Can you work these out from the model? Positions are in its coordinate system, mm. A direction names the side the tool comes from. Round coordinates to 2 decimals unless told otherwise and drop trailing zeros. Order: outer loops, then holes, each group sorted by start corner. A loop starts at its lowest first (then second) coordinate and runs counter-clockwise, first axis right, second up. Notation, with made-up numbers: (29, 75) -> (53, 75) arc R33 cw to (53, 103) -> close; hole circle Ø9 at (64, 8.25). An arc over 180 degrees is marked (long way). Use a Markdown table: item, result. Add a question column.
Q1. I need wall thicknesses on line 1 along Z through (x, y) = (-62, 4.2); line 2 along X through (y, z) = (1.65, -12.5); line 3 along X through (y, z) = (1.45, -61). Which ranges of each line are inside material? Lowest first, please. Write a range as [from, to].
Q2. If we section it at D-D on x = -42: List the corners of the cut face in (y, z) for me, plus the area to 3 significant figures.
Q3. If we section it at A-A on z = -37.5: List the corners of the cut face in (x, y) for me, plus the area to 3 significant figures.
Q4. If we section it at B-B on x = -87: List the corners of the cut face in (y, z) for me, plus the area to 3 significant figures.
Q5. We'd pull the mould along X, two halves only. Please class faces 1 (the face through (-44.027, 3.042, -39.359)), 2 (the face through (-103, 3, -74)), 3 (the face through (-33, 3, -2)): +X half, -X half, draft (parallel to the pull), parting line (faces both ways), or undercut.
Q6. If we section it at C-C on y = 1.65: List the corners of the cut face in (x, z) for me.
Q7. For faces 4 (the face through (-75, 3, -62)), 5 (the face through (-105, 3, -37)), 6 (the face through (-84.25, 3, -65)), which set-ups out of +Z, -Z, +X, -X, +Y, -Y let a thin tool reach every point of the face, with its end or its side?
Q8. I'm going to push flat-ended pins straight in: pin 1 Ø5 at (x, z) = (-62, -37.5) entering from +Y; pin 2 Ø3 at (y, z) = (3, -61) entering from +X. Where does each tip first touch, or does it pass through?
Autodesk Inventor part; units mm, degrees
ref_plane "YZ Plane" through (0, 0, 0) normal (1, 0, 0) x (0, 1, 0)
ref_plane "XZ Plane" through (0, 0, 0) normal (0, 1, 0) x (-1, 0, 0)
ref_plane "XY Plane" through (0, 0, 0) normal (0, 0, 1) x (1, 0, 0)
sketch "Sketch1" plane through (0, 0, 0) normal (0, 1, 0) x (-1, 0, 0)
  line L0 (0, 0) -> (105, 0)
  line L1 (105, 0) -> (105, -50)
  line L2 (105, -50) -> (0, -50)
  line L3 (0, -50) -> (0, 0)
  line L4 (0, 0) -> (0, -16.6667)
  line L5 (0, -16.6667) -> (11, -16.6667)
  dimension "d0" = 105
  dimension "d1" = 50
  dimension "d2" = 16.6667
  dimension "d3" = 11
extrude "Extrusion1" add sketch "Sketch1" along normal blind 6
sketch "Sketch3" plane through (0, 6, 0) normal (0, 1, 0) x (1, 0, 0)
  circle A0 centre (-20, 12.5) radius 2.75
  line L0 (0, 0) -> (0, 50)
  line L1 (-105, 0) -> (0, 0)
  circle A1 centre (-20, 37.5) radius 2.75
  dimension "d21" = 5.5
  dimension "d22" = 20
  dimension "d23" = 12.5
  dimension "d26" = 25
extrude "Extrusion3" cut sketch "Sketch3" against normal through all
sketch "Sketch4" plane through (0, 6, 0) normal (0, 1, 0) x (1, 0, 0)
  circle A0 centre (-20, 12.5) radius 2.75
  line L0 (-20, 12.5) -> (-75, 12.5)
  line L1 (-75, 12.5) -> (-90, 12.5) construction
  line L2 (-75, 15.25) -> (-90, 15.25)
  line L3 (-90, 9.75) -> (-75, 9.75)
  arc A1 (-75, 9.75) -> (-75, 15.25) centre (-75, 12.5) ccw
  arc A2 (-90, 15.25) -> (-90, 9.75) centre (-90, 12.5) ccw
  point P0 (0, 0)
  point P1 (-82.5, 12.5)
  dimension "d33" = 55
  dimension "d34" = 15
  dimension "d35" = 5.5
extrude "Extrusion4" cut sketch "Sketch4" against normal through all contours A1 L3 A2 L2
pattern_linear "Rectangular Pattern2" count 2 spacing 25 along (0, 0, -1) of "Extrusion4"
sketch "Sketch5" plane through (0, 0, -50) normal (0, 0, -1) x (-1, 0, 0)
  line L0 (105, 0) -> (105, 6)
  line L1 (105, 0) -> (0, 0)
  line L2 (105, 6) -> (75, 6)
  line L3 (75, 6) -> (75, 0)
  line L4 (75, 0) -> (105, 0)
  line L5 (105, 0) -> (105, 6)
  dimension "d45" = 30
extrude "Extrusion5" add sketch "Sketch5" along normal blind 25
sketch "Sketch6" plane through (0, 6, 0) normal (0, 1, 0) x (1, 0, 0)
  line L0 (-87, 60.5) -> (-87, 70.5) construction
  line L1 (-84.25, 60.5) -> (-84.25, 70.5)
  line L2 (-89.75, 70.5) -> (-89.75, 60.5)
  arc A0 (-89.75, 60.5) -> (-84.25, 60.5) centre (-87, 60.5) ccw
  arc A1 (-84.25, 70.5) -> (-89.75, 70.5) centre (-87, 70.5) ccw
  line L3 (-75, 50) -> (-75, 75)
  arc A2 (-90, 40.25) -> (-90, 34.75) centre (-90, 37.5) ccw
  point P0 (0, 0)
  point P1 (-87, 65.5)
  dimension "d48" = 10
  dimension "d49" = 5.5
  dimension "d50" = 12
  dimension "d51" = 28
extrude "Extrusion6" cut sketch "Sketch6" against normal through all
fillet "Fillet2" radius 5 6 edges at (-105, 3, 0) (0, 3, 0) (-75, 3, -75) (-105, 3, -75) (0, 3, -50) (-75, 3, -50)
sketch "Sketch7" plane through (0, 6, 0) normal (0, 1, 0) x (1, 0, 0)
  circle A0 centre (-20, 12.5) radius 2.75
  line L0 (-20, 12.5) -> (-42, 12.5)
  line L1 (-42, 12.5) -> (-62, 12.5)
  circle A1 centre (-62, 12.5) radius 2.75
  circle A2 centre (-42, 12.5) radius 2.75
  line L2 (0, 5) -> (0, 45)
  line L3 (0, 0) -> (0, 45)
  circle A3 centre (-42, 37.5) radius 2.75
  circle A4 centre (-62, 37.5) radius 2.75
  dimension "d55" = 22
  dimension "d56" = 20
  dimension "d57" = 5.5
  dimension "d58" = 5.5
  dimension "d61" = 25
extrude "Extrusion7" cut sketch "Sketch7" against normal through all contours A2 L1 L0 | L0 L1 A2 | A1 | A3 | A4
sketch "Sketch9" plane through (0, 6, 0) normal (0, 1, 0) x (1, 0, 0)
  point P0 (0, 0)
sketch "Sketch12" plane through (0, 6, 0) normal (0, 1, 0) x (1, 0, 0)
  circle A0 centre (-42, 37.5) radius 2.75
  line L0 (-42, 37.5) -> (-32, 37.5)
  line L1 (-32, 37.5) -> (-32, 50)
  line L2 (-5, 50) -> (-70, 50)
  line L3 (-32, 50) -> (0, 50)
  line L4 (0, 50) -> (0, 0)
  line L5 (0, 0) -> (-32, 0)
  line L6 (-32, 0) -> (-32, 50)
  dimension "d87" = 10
extrude "Extrusion10" cut sketch "Sketch12" against normal blind 10 contours L1 L2 L3 L4 L5 L6
fillet "Fillet3" radius 5 2 edges at (-32, 3, 0) (-32, 3, -50)
properties part number "X_Carriage_Plate_Short"
Answer below:
| question | item | result |
|---|---|---|
| 1 | line 1 | [-50, -40.25], [-34.75, -15.25], [-9.75, 0] |
| 1 | line 2 | [-105, -92.75], [-72.25, -64.75], [-59.25, -44.75], [-39.25, -32] |
| 1 | line 3 | [-105, -89.75], [-84.25, -75] |
| 2 | outline | (0, -50) -> (6, -50) -> (6, -40.25) -> (0, -40.25) -> close; (0, -34.75) -> (6, -34.75) -> (6, -15.25) -> (0, -15.25) -> close; (0, -9.75) -> (6, -9.75) -> (6, 0) -> (0, 0) -> close |
| 2 | area | 234 mm² |
| 3 | outline | (-105, 0) -> (-92.75, 0) -> (-92.75, 6) -> (-105, 6) -> close; (-72.25, 0) -> (-64.75, 0) -> (-64.75, 6) -> (-72.25, 6) -> close; (-59.25, 0) -> (-44.75, 0) -> (-44.75, 6) -> (-59.25, 6) -> close; (-39.25, 0) -> (-32, 0) -> (-32, 6) -> (-39.25, 6) -> close |
| 3 | area | 249 mm² |
| 4 | outline | (0, -75) -> (6, -75) -> (6, -73.25) -> (0, -73.25) -> close; (0, -57.75) -> (6, -57.75) -> (6, -40.25) -> (0, -40.25) -> close; (0, -34.75) -> (6, -34.75) -> (6, -15.25) -> (0, -15.25) -> close; (0, -9.75) -> (6, -9.75) -> (6, 0) -> (0, 0) -> close |
| 4 | area | 291 mm² |
| 5 | face 1 | undercut |
| 5 | face 2 | -X half |
| 5 | face 3 | +X half |
| 6 | outline | (-105, -70) arc R5 ccw to (-100, -75) -> (-80, -75) arc R5 ccw to (-75, -70) -> (-75, -55) arc R5 cw to (-70, -50) -> (-37, -50) arc R5 ccw to (-32, -45) -> (-32, -5) arc R5 ccw to (-37, 0) -> (-100, 0) arc R5 ccw to (-105, -5) -> close; hole (-90, -40.25) -> (-75, -40.25) arc R2.75 ccw to (-75, -34.75) -> (-90, -34.75) arc R2.75 ccw to start; hole (-90, -15.25) -> (-75, -15.25) arc R2.75 ccw to (-75, -9.75) -> (-90, -9.75) arc R2.75 ccw to start; hole (-89.75, -70.5) arc R2.75 ccw to (-84.25, -70.5) -> (-84.25, -60.5) arc R2.75 ccw to (-89.75, -60.5) -> close; hole circle Ø5.5 at (-62, -37.5); hole circle Ø5.5 at (-62, -12.5); hole circle Ø5.5 at (-42, -37.5); hole circle Ø5.5 at (-42, -12.5) |
| 7 | face 4 | -Z, +X, +Y, -Y |
| 7 | face 5 | +Z, -Z, -X, +Y, -Y |
| 7 | face 6 | +Y, -Y |
| 8 | pin 1 | through |
| 8 | pin 2 | x = -75 |
